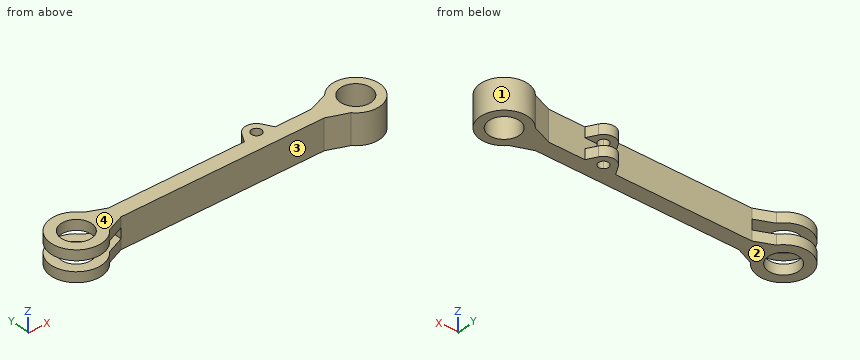
from build123d import *

# Parameters (mm, degrees)
SKETCH1_R           = 30
BOSS_EXTRUDE1_DEPTH = 60
SKETCH2_W           = 125
SKETCH2_H           = 20
CUT_EXTRUDE1_DEPTH  = 70
BOSS_EXTRUDE2_DEPTH = 60
SKETCH4_R           = 10
CUT_EXTRUDE2_DEPTH  = 61
SKETCH5_W           = 20
SKETCH5_H           = 30.196617065
CUT_EXTRUDE3_DEPTH  = 350


with BuildPart() as part:
    # Sketch1 → Boss-Extrude1 (new body)
    with BuildSketch(Plane.XY):
        with BuildLine():
            Line((200, 15), (-200, 15))
            Line((-200, 15), (-234.992965725, 30.413109921))
            ThreePointArc((-234.992965725, 30.413109921), (-325, 0.422491245), (-234.992965725, -29.568127431))
            Line((-234.992965725, -29.568127431), (-200, -15))
            Line((-200, -15), (200, -15))
            Line((200, -15), (239.447282721, -30.416066909))
            ThreePointArc((239.447282721, -30.416066909), (321.788169788, 0), (239.447282721, 30.416066909))
            Line((239.447282721, 30.416066909), (200, 15))
        make_face()
        with Locations((-275, 0.422491245)):
            Circle(SKETCH1_R, mode=Mode.SUBTRACT)
        with Locations((275, 0)):
            Circle(SKETCH1_R, mode=Mode.SUBTRACT)
    extrude(amount=BOSS_EXTRUDE1_DEPTH)

    # Sketch2 → Cut-Extrude1 (cut, symmetric)
    with BuildSketch(Plane(origin=(0, 15, 0), x_dir=(1, 0, 0), z_dir=(0, 1, 0))):
        with Locations((-262.5, -30)):
            Rectangle(SKETCH2_W, SKETCH2_H)
    extrude(amount=CUT_EXTRUDE1_DEPTH, both=True, mode=Mode.SUBTRACT)

    # Sketch3 → Boss-Extrude2 (add)
    with BuildSketch(Plane.XY.offset(60)):
        with BuildLine():
            ThreePointArc((118.204825436, 33.881006124), (98.681520352, 45.196617065), (79.158215269, 33.881006124))
            ThreePointArc((79.158215269, 33.881006124), (76.263820119, 24.619301704), (77.538860024, 15))
            Line((77.538860024, 15), (92.297001125, 15))
            ThreePointArc((92.297001125, 15), (98.681520352, 32.696617065), (105.066039579, 15))
            Line((105.066039579, 15), (119.824180681, 15))
            ThreePointArc((119.824180681, 15), (121.099220586, 24.619301704), (118.204825436, 33.881006124))
        make_face()
        with BuildLine():
            ThreePointArc((77.538860024, 15), (76.263820119, 24.619301704), (79.158215269, 33.881006124))
            Line((79.158215269, 33.881006124), (68.341782426, 15))
            Line((68.341782426, 15), (77.538860024, 15))
        make_face()
        with BuildLine():
            Line((129.021258279, 15), (118.204825436, 33.881006124))
            ThreePointArc((118.204825436, 33.881006124), (121.099220586, 24.619301704), (119.824180681, 15))
            Line((119.824180681, 15), (129.021258279, 15))
        make_face()
    extrude(amount=-BOSS_EXTRUDE2_DEPTH)

    # Sketch4 → Cut-Extrude2 (cut, through all)
    with BuildSketch(Plane.XY.offset(60)):
        with Locations((98.681520352, 22.696617065)):
            Circle(SKETCH4_R)
    extrude(amount=-CUT_EXTRUDE2_DEPTH, mode=Mode.SUBTRACT)

    # Sketch5 → Cut-Extrude3 (cut)
    with BuildSketch(Plane.ZY.offset(200)):
        with Locations((30, 30.098308533)):
            Rectangle(SKETCH5_W, SKETCH5_H)
    extrude(amount=-CUT_EXTRUDE3_DEPTH, mode=Mode.SUBTRACT)


solid = part.part
Input: part model. Units: mm. Frame: model coordinates. Face numbers are marked on the shaded views. A direction names the side the tool comes from. Coordinates: 2 decimals unless noted, no trailing zeros. Loops run counter-clockwise (first coordinate to the right, second up) from the corner with the lowest first, then second, coordinate; pieces in that order, holes last.
(1) Set-up query: the marked faces 3 and 4. Return all of +Z, -Z, +X, -X, +Y, -Y with unobstructed straight access to the full face (end or side cutting, diameter ignored); none if empty.
(2) Section D-D on x = -132. Return the cut outline in (y, z), then the cut area to 3 significant figures.
(3) Material intervals for probe 1 along Y at (x, z) = (275, 22); probe 2 along Y at (x, z) = (-275, 12.5); probe 3 along X at (y, z) = (-11, 15), sorted ascending.
(4) Section A-A on x = -275. Return the cut outline in (y, z), then the cut area to 3 significant figures.
(5) Section C-C on z = 34.5. Return the cut outline in (x, y), then the cut area to 3 significant figures.
(6) Section B-B on x = 275. Return the cut outline in (y, z), then the cut area to 3 significant figures.
(7) First-contact query: pin 1 Ø4 at (x, z) = (-28, 23) entering from -Y; pin 2 Ø3 at (y, z) = (40.5, 32.5) entering from -X; pin 3 Ø5 at (y, z) = (-12, 23) entering from +X. Flat tips, straight axial feed; report the tip coordinate or a pass-through.
(8) Pull-direction query (X, two-part tool) for the marked faces 1 and 2; classes: released by +X, released by -X, zero draft, split by the parting line, or undercut.
Data:
1. face 3: +Z, -Z, -Y
1. face 4: +Z, +X, -X, +Y, -Y
2. outline: (-15, 0) - (15, 0) - (15, 60) - (-15, 60) - close
2. area: 1,800 mm2
3. probe 1: y = -46.79 to -30, 30 to 46.79
3. probe 2: y = -49.58 to -29.58, 30.42 to 50.42
3. probe 3: x = -323.68 to -302.74, -247.26 to 247.09, 302.91 to 320.48
4. outline: (-49.58, 0) - (-29.58, 0) - (-29.58, 20) - (-49.58, 20) - close; (-49.58, 40) - (-29.58, 40) - (-29.58, 60) - (-49.58, 60) - close; (30.42, 0) - (50.42, 0) - (50.42, 20) - (30.42, 20) - close; (30.42, 40) - (50.42, 40) - (50.42, 60) - (30.42, 60) - close
4. area: 1,600 mm2
5. outline: (-200, -15) - (200, -15) - (239.45, -30.42) arc R46.79 ccw (long way) to (239.45, 30.42) - (200, 15) - (105.07, 15) arc R10 cw to (92.3, 15) - (-200, 15) - close; hole circle Ø60 at (275, 0)
5. area: 17,400 mm2
6. outline: (-46.79, 0) - (-30, 0) - (-30, 60) - (-46.79, 60) - close; (30, 0) - (46.79, 0) - (46.79, 60) - (30, 60) - close
6. area: 2,010 mm2
7. pin 1: stops at y = -15
7. pin 2: stops at x = 249.15
7. pin 3: stops at x = 320.81
8. face 1: undercut
8. face 2: zero draft
